from build123d import *

# Parameters (mm, degrees)
F3_DEPTH = 25.4


with BuildPart() as f1:
    # F0 (on Front) → F1 (revolve)
    with BuildSketch(Plane.XZ):
        Polygon((-12.7635, 0), (0, 0), (0, 12.7), (-12.1285, 12.7), (-12.7635, 12.7), align=None)
        Polygon((-12.7635, 12.7), (-12.1285, 12.7), (-12.7635, 13.335), align=None)
    revolve(axis=Axis((0, 0, 6.35), (0, 0, 1)))

    # F2 (on face) → F3 (join)
    with BuildSketch(Plane(origin=(0, 0, 0), x_dir=(1, 0, 0), z_dir=(0, 0, -1))):
        with BuildLine():
            Line((10.191701, 7.6835), (-10.191701, 7.6835))
            ThreePointArc((-10.191701, 7.6835), (0, -12.7635), (10.191701, 7.6835))
        make_face()
    extrude(amount=F3_DEPTH)


solid = f1.part
Build history of the part. All positions in model axes, mm. Coordinates: 2 decimals unless noted, no trailing zeros. Order: outer loops, then holes, each group sorted by start corner. A loop starts at its lowest first (then second) coordinate and runs counter-clockwise, first axis right, second up. Notation, with made-up numbers: M -5,-30 L 5,-30 A29 ccw 5,7 Z; hole C -14.5,6 d1. An arc over 180 degrees is marked long. One line per question, with ' | ' between items. Start each with the question number.
Q1. Probe L1, parallel to Z at x = -4, y = 10.75; L2, parallel to Y at x = -0.5, z = 10; L3, parallel to Z at x = -2.75, y = -10.25. List the from-to ranges inside material, lowest first. Write a range as from..to.
Q2. Two-plate mould, pull along Y, no slides. Class faces 1 (the face through (0, 0, 12.7)), 2 (the face through (0, -7.684, -13)), 3 (the face through (0, -10, 0)): +Y half, -Y half, draft (parallel to the pull), parting line (faces both ways), or undercut.
Q3. Saw through at C-C (z = -9). List the corners of the cut face in (x, y).
Q4. Flat gauge pins, fed straight in: pin 1 Ø1 at (x, y) = (-0.5, 4.5) entering from +Z; pin 2 Ø4 at (y, z) = (-8.5, -20.5) entering from +X; pin 3 Ø3 at (x, z) = (1.5, -18) entering from -Y. Where does each tip first touch, or does it go through?
Q5. Saw through at D-D (z = 0.5). List the corners of the cut face in (x, y).
Q6. Saw through at A-A (x = 0). List the corners of the cut face in (y, z) (1 decimal).
Q7. Saw through at B-B (y = 0). List the corners of the cut face in (x, z) (1 decimal), then the cut area to 3 significant figures.
Check values:
1) L1: z = -25.4..12.7 | L2: y = -12.75..12.75 | L3: z = 0..12.7
2) face 1: undercut | face 2: -Y half | face 3: draft
3) outline: M -10.19,-7.68 L 10.19,-7.68 A12.76 ccw long Z
4) pin 1: stops at z = 12.7 | pin 2: stops at x = 10.98 | pin 3: stops at y = -7.68
5) outline: C 0,0 d25.53
6) outline: M -12.8,0 L -7.7,0 L -7.7,-25.4 L 12.8,-25.4 L 12.8,13.3 L 12.1,12.7 L -12.1,12.7 L -12.8,13.3 Z
7) outline: M -12.8,-25.4 L 12.8,-25.4 L 12.8,13.3 L 12.1,12.7 L -12.1,12.7 L -12.8,13.3 Z | area: 973 mm2
